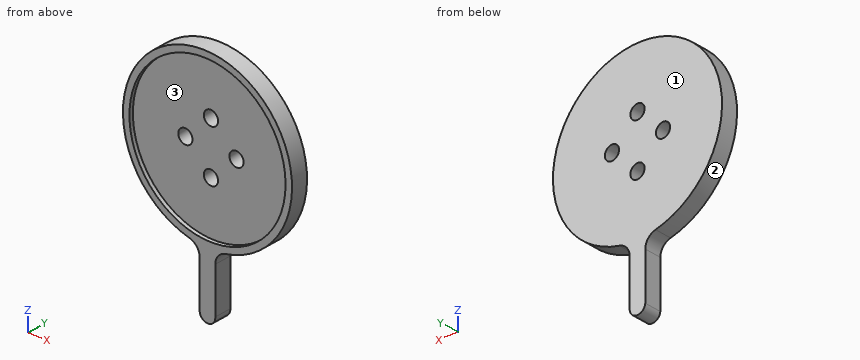
```python
from build123d import *

# Parameters (mm, degrees)
SKETCH2_R           = 32.76798012
BOSS_EXTRUDE1_DEPTH = 5
SKETCH3_R           = 32.76798012
SKETCH3_R_2         = 30.26798012
BOSS_EXTRUDE2_DEPTH = 1.5
SKETCH4_R           = 2.75
CUT_EXTRUDE1_DEPTH  = 9.8994949
BOSS_EXTRUDE3_DEPTH = 6.5


with BuildPart() as part:
    # Sketch2 → Boss-Extrude1 (new body)
    with BuildSketch(Plane(origin=(0, 0, 0), x_dir=(1, 0, 0), z_dir=(0, 1, 0))):
        Circle(SKETCH2_R)
    extrude(amount=BOSS_EXTRUDE1_DEPTH)

    # Sketch3 → Boss-Extrude2 (add)
    with BuildSketch(Plane.XZ):
        Circle(SKETCH3_R)
        Circle(SKETCH3_R_2, mode=Mode.SUBTRACT)
    extrude(amount=BOSS_EXTRUDE2_DEPTH)

    # Sketch4 → Cut-Extrude1 (cut)
    with BuildSketch(Plane(origin=(0, 5, 0), x_dir=(1, 0, 0), z_dir=(0, 1, 0))):
        with Locations((0, 9.8994949)):
            Circle(SKETCH4_R)
        with Locations((-9.9, 0)):
            Circle(SKETCH4_R)
        with Locations((9.9, 0)):
            Circle(SKETCH4_R)
        with Locations((0, -9.9)):
            Circle(SKETCH4_R)
    extrude(amount=-CUT_EXTRUDE1_DEPTH, mode=Mode.SUBTRACT)

    # Sketch5 → Boss-Extrude3 (add)
    with BuildSketch(Plane(origin=(0, 5, 0), x_dir=(1, 0, 0), z_dir=(0, 1, 0))):
        with BuildLine():
            Line((-3.023415672, 36.951680319), (-3.023415672, 54.951680319))
            ThreePointArc((-3.023415672, 54.951680319), (0.237235199, 57.737860793), (3.023415672, 54.477209922))
            Line((3.023415672, 54.477209922), (3.023415672, 36.951680319))
            ThreePointArc((3.023415672, 36.951680319), (4.141073493, 33.780800032), (7, 32.011568552))
            ThreePointArc((7, 32.011568552), (0, 32.76798012), (-7, 32.011568552))
            ThreePointArc((-7, 32.011568552), (-4.141073493, 33.780800032), (-3.023415672, 36.951680319))
        make_face()
    extrude(amount=-BOSS_EXTRUDE3_DEPTH)


solid = part.part
```
Geometry check sheet. Reference: the model listing, model coordinates, mm. Face numbers are marked on the shaded views. Round coordinates to 2 decimals unless told otherwise and drop trailing zeros. Order: outer loops, then holes, each group sorted by start corner. A loop starts at its lowest first (then second) coordinate and runs counter-clockwise, first axis right, second up. Notation, with made-up numbers: (20.25, 18.5) - (40.25, 18.5) arc R16 ccw to (40.25, 39.5) - close; hole circle Ø6 at (24, 80). An arc over 180 degrees is marked (long way). Use a Markdown table: item, result. Add a question column.
1) Section check A-A (x = -9.9). Record the cut outline in (y, z), then the cut area to 3 significant figures.
2) Section check D-D (y = 2.5). Record the cut outline in (x, z), then the cut area to 3 significant figures.
3) Section check B-B (z = 0). Record the cut outline in (x, y).
4) Section check C-C (x = 0). Record the cut outline in (y, z).
5) Mould release check, pull along X, two halves, no side actions. Record for the marked faces 1, 2 and 3: released by +X, released by -X, zero draft, split by the parting line, or undercut.
6) Gauge pin test, flat ends, axial feed: P1, Ø1, axis at x = -11, y = -0.5, coming from the -Z side; P2, Ø18, axis at x = 11, z = -3.5, coming from the -Y side; P3, Ø3, axis at y = -0.5, z = 4, coming from the +X side. Record the tip position at first contact, or that the pin passes through.
7) Thickness scan on line 1 along X through (y, z) = (1.8, 0); line 2 along Z through (x, y) = (0, -0.9); line 3 along Z through (x, y) = (0, 1.85). Record the ranges inside material, lowest first.
Established:
| question | item | result |
|---|---|---|
| 1 | outline | (-1.5, -31.24) - (5, -31.24) - (5, -2.75) - (0, -2.75) - (0, -28.6) - (-1.5, -28.6) - close; (-1.5, 28.6) - (0, 28.6) - (0, 2.75) - (5, 2.75) - (5, 31.24) - (-1.5, 31.24) - close |
| 1 | area | 293 mm2 |
| 2 | outline | (-7, -32.01) arc R5.06 cw to (-3.02, -36.95) - (-3.02, -54.95) arc R3.03 ccw to (3.02, -54.48) - (3.02, -36.95) arc R5.06 cw to (7, -32.01) arc R32.77 ccw (long way) to start; hole circle Ø5.5 at (-9.9, 0); hole circle Ø5.5 at (0, -9.9); hole circle Ø5.5 at (0, 9.9); hole circle Ø5.5 at (9.9, 0) |
| 2 | area | 3,430 mm2 |
| 3 | outline | (-32.77, -1.5) - (-30.27, -1.5) - (-30.27, 0) - (-12.65, 0) - (-12.65, 5) - (-32.77, 5) - close; (-7.15, 0) - (7.15, 0) - (7.15, 5) - (-7.15, 5) - close; (12.65, 0) - (30.27, 0) - (30.27, -1.5) - (32.77, -1.5) - (32.77, 5) - (12.65, 5) - close |
| 4 | outline | (-1.5, -57.75) - (5, -57.75) - (5, -12.65) - (0, -12.65) - (0, -30.27) - (-1.5, -30.27) - close; (-1.5, 30.27) - (0, 30.27) - (0, 12.65) - (5, 12.65) - (5, 32.77) - (-1.5, 32.77) - close; (0, -7.15) - (5, -7.15) - (5, 7.15) - (0, 7.15) - close |
| 5 | face 1 | zero draft |
| 5 | face 2 | split by the parting line |
| 5 | face 3 | undercut |
| 6 | P1 | z = -31.04 |
| 6 | P2 | y = 0 |
| 6 | P3 | x = 32.67 |
| 7 | line 1 | -32.77 to -12.65, -7.15 to 7.15, 12.65 to 32.77 |
| 7 | line 2 | -57.75 to -30.27, 30.27 to 32.77 |
| 7 | line 3 | -57.75 to -12.65, -7.15 to 7.15, 12.65 to 32.77 |
